CAD build for the part. Positions are in the model's coordinates, mm. A direction names the side the tool comes from. Coordinates: 2 decimals unless noted, no trailing zeros. Loops run counter-clockwise (first coordinate to the right, second up) from the corner with the lowest first, then second, coordinate; pieces in that order, holes last. Notation, with made-up numbers: (-11.75, 84.25) -> (19.25, 84.25) arc R10 cw to (19.25, 95.25) -> close; hole circle Ø9 at (45.25, 22). An arc over 180 degrees is marked (long way). Write item = value, one per line. Start each with the question number.
(1) Band-saw the part on D-D (y = 2.45). Count the separate pieces of the cut face and the enclosed holes in it, and give its area (3 significant figures).
(2) Band-saw the part on B-B (z = -4.5). Write the cut outline in (x, y).
(3) Pull direction X, two halves, no side cores. Call faces 1 (the face through (-25.861, 1.479, -33.727)), 2 (the face through (16.98, 1.52, -16.25)), 3 (the face through (-18, 3, 18)): +X half, -X half, draft (parallel to the pull), parting line (faces both ways), or undercut.
(4) Band-saw the part on A-A (x = 0). Write the cut outline in (y, z), and give its area (3 significant figures).
(5) Drill centre lines: line 1 (Z direction, x = 0.5, y = 2.85); line 2 (X direction, y = 2.55, z = 21); line 3 (X direction, y = 2.6, z = 18.5). Where is each one in solid material? Low to high. Write a range as from..to.
(6) Flat gauge pin, fed straight in: P1, Ø4, axis at x = 20.5, z = 19.8, coming from the +Y side. Where does the tip first touch, or does it go through?
(7) Band-saw the part on C-C (x = 20.5). Write the cut outline in (y, z).
(8) Tool access for faces 4 (the face through (-0.2, 1.5, 32.5)), 5 (the face through (-18, 0, 18)): list every direction of +Z, -Z, +X, -X, +Y, -Y with a clear straight run to the whole face (end or side of a thin tool).
```python
from build123d import *

# Parameters (mm, degrees)
SKETCH_1_R          = 45
SKETCH_1_R_2        = 2
EXTRUDE_1_DEPTH     = 3
CUT_EXTRUDE_1_DEPTH = 64.710281745
FILLET_1_R          = 3
MOVE_FACE_1_BY      = 2.5
MOVE_FACE_2_BY      = 0.15
MOVE_FACE_2_2_BY    = 0.15
MOVE_FACE_2_3_BY    = 0.15
MOVE_FACE_2_4_BY    = 0.15
MOVE_FACE_3_BY      = 0.4
MOVE_FACE_3_2_BY    = 0.4
MOVE_FACE_3_3_BY    = 0.4
MOVE_FACE_3_4_BY    = 0.4


with BuildPart() as part:
    # ｽｹｯﾁ1 → ﾎﾞｽ - 押し出し1 (new body)
    with BuildSketch(Plane(origin=(0, 0, 0), x_dir=(1, 0, 0), z_dir=(0, 1, 0))):
        with Locations(Location((0, 0, 0), (0, 0, 270))):
            Circle(SKETCH_1_R)
        with Locations(Location((-20.5, -19.798989873, 0), (0, 0, 270))):
            Circle(SKETCH_1_R_2, mode=Mode.SUBTRACT)
        with Locations(Location((20.5, -19.798989873, 0), (0, 0, 90))):
            Circle(SKETCH_1_R_2, mode=Mode.SUBTRACT)
        with Locations(Location((20.5, 19.798989873, 0), (0, 0, 270))):
            Circle(SKETCH_1_R_2, mode=Mode.SUBTRACT)
        with Locations(Location((-20.5, 19.798989873, 0), (0, 0, 90))):
            Circle(SKETCH_1_R_2, mode=Mode.SUBTRACT)
    extrude(amount=EXTRUDE_1_DEPTH)

    # ｽｹｯﾁ2 → ｶｯﾄ - 押し出し1 (cut, through all)
    with BuildSketch(Plane(origin=(0, 3, 0), x_dir=(1, 0, 0), z_dir=(0, 1, 0))):
        with BuildLine():
            ThreePointArc((25.486471606, -20.166550649), (30.696582279, -10.675665619), (32.5, 0))
            ThreePointArc((32.5, 0), (30.696582279, 10.675665619), (25.486471606, 20.166550649))
            ThreePointArc((25.486471606, 20.166550649), (25.496616757, 19.9828947), (25.5, 19.798989873))
            ThreePointArc((25.5, 19.798989873), (16.778183392, 16.460115641), (21.040767545, 24.769660901))
            ThreePointArc((21.040767545, 24.769660901), (0, 32.5), (-21.040767545, 24.769660901))
            ThreePointArc((-21.040767545, 24.769660901), (-17.161125768, 23.520806481), (-15.5, 19.798989873))
            ThreePointArc((-15.5, 19.798989873), (-20.683904827, 14.802373116), (-25.486471606, 20.166550649))
            ThreePointArc((-25.486471606, 20.166550649), (-32.5, 0), (-25.486471606, -20.166550649))
            ThreePointArc((-25.486471606, -20.166550649), (-20.683904827, -14.802373116), (-15.5, -19.798989873))
            ThreePointArc((-15.5, -19.798989873), (-17.161125768, -23.520806481), (-21.040767545, -24.769660901))
            ThreePointArc((-21.040767545, -24.769660901), (0, -32.5), (21.040767545, -24.769660901))
            ThreePointArc((21.040767545, -24.769660901), (16.778183392, -16.460115641), (25.5, -19.798989873))
            ThreePointArc((25.5, -19.798989873), (25.496616757, -19.9828947), (25.486471606, -20.166550649))
        make_face()
    extrude(amount=-CUT_EXTRUDE_1_DEPTH, mode=Mode.SUBTRACT)

    # ﾌｨﾚｯﾄ1
    fillet_1_edges = [part.edges().sort_by_distance(p)[0] for p in [
        (21.040767545, 1.5, -24.769660901),
        (25.486471606, 1.5, -20.166550649),
        (25.486471606, 1.5, 20.166550649),
        (21.040767545, 1.5, 24.769660901),
        (-21.040767545, 1.5, 24.769660901),
        (-25.486471606, 1.5, 20.166550649),
        (-25.486471606, 1.5, -20.166550649),
        (-21.040767545, 1.5, -24.769660901),
    ]]
    fillet(fillet_1_edges, radius=FILLET_1_R)

    # Move Face 1: a curved face moved inward by 2.5
    add(Solid.thicken(part.faces().sort_by_distance((0, 1.5, -45))[0], -MOVE_FACE_1_BY), mode=Mode.SUBTRACT)

    # Move Face 2: a curved face moved inward by 0.15
    add(Solid.thicken(part.faces().sort_by_distance((20.5, 1.5, -21.798989873))[0], -MOVE_FACE_2_BY), mode=Mode.SUBTRACT)

    # Move Face 2 2: a curved face moved inward by 0.15
    add(Solid.thicken(part.faces().sort_by_distance((-20.5, 1.5, -17.798989873))[0], -MOVE_FACE_2_2_BY), mode=Mode.SUBTRACT)

    # Move Face 2 3: a curved face moved inward by 0.15
    add(Solid.thicken(part.faces().sort_by_distance((-20.5, 1.5, 17.798989873))[0], -MOVE_FACE_2_3_BY), mode=Mode.SUBTRACT)

    # Move Face 2 4: a curved face moved inward by 0.15
    add(Solid.thicken(part.faces().sort_by_distance((20.5, 1.5, 21.798989873))[0], -MOVE_FACE_2_4_BY), mode=Mode.SUBTRACT)

    # Move Face 3: a curved face moved outward by 0.4
    add(Solid.thicken(part.faces().sort_by_distance((-20.5, 1.5, 17.648989873))[0], MOVE_FACE_3_BY))

    # Move Face 3 2: a curved face moved outward by 0.4
    add(Solid.thicken(part.faces().sort_by_distance((20.5, 1.5, 21.948989873))[0], MOVE_FACE_3_2_BY))

    # Move Face 3 3: a curved face moved outward by 0.4
    add(Solid.thicken(part.faces().sort_by_distance((20.5, 1.5, -21.948989873))[0], MOVE_FACE_3_3_BY))

    # Move Face 3 4: a curved face moved outward by 0.4
    add(Solid.thicken(part.faces().sort_by_distance((-20.5, 1.5, -17.648989873))[0], MOVE_FACE_3_4_BY))


solid = part.part
```
Findings below:
q1.separate_pieces = 1
q1.enclosed_holes = 5
q1.area = 2,660 mm²
q2.outline = (-42.26, 0) -> (-32.19, 0) -> (-32.19, 3) -> (-42.26, 3) -> close; (32.19, 0) -> (42.26, 0) -> (42.26, 3) -> (32.19, 3) -> close
q3.face_1 = parting line
q3.face_2 = undercut
q3.face_3 = draft
q4.outline = (0, -42.5) -> (3, -42.5) -> (3, -32.5) -> (0, -32.5) -> close; (0, 32.5) -> (3, 32.5) -> (3, 42.5) -> (0, 42.5) -> close
q4.area = 60.0 mm²
q5.line_1 = -42.5..-32.5, 32.5..42.5
q5.line_2 = -36.95..-21.77, -19.23..-15.65, 15.65..19.23, 21.77..36.95
q5.line_3 = -38.26..-21.67, -19.33..-15.67, 15.67..19.33, 21.67..38.26
q6.P1 = 3
q7.outline = (0, -37.23) -> (3, -37.23) -> (3, -21.55) -> (0, -21.55) -> close; (0, -18.05) -> (3, -18.05) -> (3, -14.8) -> (0, -14.8) -> close; (0, 14.8) -> (3, 14.8) -> (3, 18.05) -> (0, 18.05) -> close; (0, 21.55) -> (3, 21.55) -> (3, 37.23) -> (0, 37.23) -> close
q8.face_4 = +Y, -Y
q8.face_5 = +Z, -Z, +X, -X, -Y
